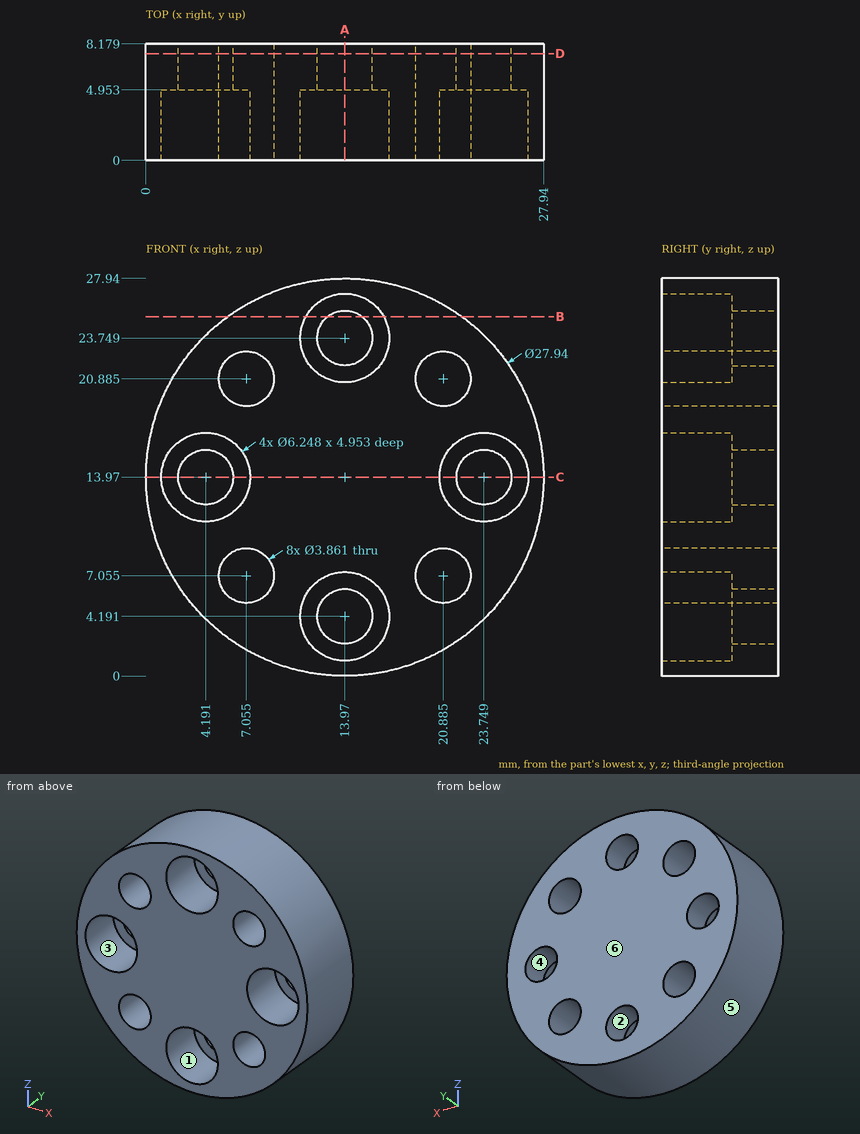
Here's the drawing with two shaded views (mm, measured from the low corner). I have some questions. A direction names the side the tool comes from. Give positions to 0.01 mm unless a question says otherwise; leave off trailing zeros. Write each loop counter-clockwise with the first axis right and the second up, starting at its lowest first coordinate (ties: lowest second). Pieces come first, ordered by that corner, then holes. Notation, with made-up numbers: (44.5, -28) -> (54.5, -28) arc R12 cw to (54.5, -13) -> close; hole circle Ø3 at (38.5, -33). An arc over 180 degrees is marked (long way). Use one line per item in the form item = value. Start each with the question number.
1. Imagine slicing it at A-A on x = 13.97. List the corners of the cut face in (y, z) for me (1 decimal), plus the area to 3 significant figures.
2. If I drill on L1, parallel to Z at x = 13.97, y = 2.65 (1 decimal); L2, parallel to Z at x = 12.25, y = 7 (1 decimal); L3, parallel to Z at x = 21.75, y = 1 (1 decimal), over which ranges is the centre line in solid material (lowest first)?
3. Imagine slicing it at C-C on z = 13.97. List the corners of the cut face in (x, y) for me (1 decimal), plus the area to 3 significant figures.
4. On a 3-axis mill with a long thin cutter (end or side, diameter ignored), from which of +Z, -Z, +X, -X, +Y, -Y can I reach the whole of each face in a straight line? I mean the marked faces 1 and 2. Say none if no direction works.
5. Imagine slicing it at B-B on z = 25.25. List the corners of the cut face in (x, y) for me.
6. Imagine slicing it at D-D on y = 7.5. State how many separate pieces and enclosed holes the cut face has.
7. Will these pins go through, and if not, where does the flat tip stop? pin 1 Ø1.9 at (x, z) = (14, 3) entering from -Y; pin 2 Ø3 at (x, z) = (13.97, 4.191) entering from +Y.
8. Thinking about a two-plate mould opening in X: for the marked faces 3, 4, 5 and 6, which applies, +X half, -X half, draft (parallel to the pull), parting line (faces both ways), or undercut?
Entries:
q1.outline = (0, 0) -> (8.2, 0) -> (8.2, 2.3) -> (5, 2.3) -> (5, 1.1) -> (0, 1.1) -> close; (0, 7.3) -> (5, 7.3) -> (5, 6.1) -> (8.2, 6.1) -> (8.2, 21.8) -> (5, 21.8) -> (5, 20.6) -> (0, 20.6) -> close; (0, 26.9) -> (5, 26.9) -> (5, 25.7) -> (8.2, 25.7) -> (8.2, 27.9) -> (0, 27.9) -> close
q1.area = 142 mm²
q2.L1 = 0 to 1.1, 7.3 to 20.6, 26.9 to 27.9
q2.L2 = 0.1 to 3.3, 5.1 to 22.9, 24.6 to 27.8
q2.L3 = 2.4 to 5.3, 8.8 to 11.6, 16.4 to 19.2, 22.6 to 25.6
q3.outline = (0, 0) -> (1.1, 0) -> (1.1, 5) -> (2.3, 5) -> (2.3, 8.2) -> (0, 8.2) -> close; (6.1, 5) -> (7.3, 5) -> (7.3, 0) -> (20.6, 0) -> (20.6, 5) -> (21.8, 5) -> (21.8, 8.2) -> (6.1, 8.2) -> close; (25.7, 5) -> (26.9, 5) -> (26.9, 0) -> (27.9, 0) -> (27.9, 8.2) -> (25.7, 8.2) -> close
q3.area = 142 mm²
q4.face_1 = -Y
q4.face_2 = +Y, -Y
q5.outline = (5.73, 0) -> (11.23, 0) -> (11.23, 4.95) -> (12.76, 4.95) -> (12.76, 8.18) -> (5.73, 8.18) -> close; (15.18, 4.95) -> (16.71, 4.95) -> (16.71, 0) -> (22.21, 0) -> (22.21, 8.18) -> (15.18, 8.18) -> close
q6.separate_pieces = 1
q6.enclosed_holes = 8
q7.pin_1 = 4.95
q7.pin_2 = through
q8.face_3 = undercut
q8.face_4 = undercut
q8.face_5 = parting line
q8.face_6 = draft
